```python
from build123d import *

# Parameters (mm, degrees)
SKETCH1_R           = 49.276
BOSS_EXTRUDE1_DEPTH = 9.525
SKETCH2_R           = 47.498
BOSS_EXTRUDE2_DEPTH = 3.175
SKETCH5_R           = 3.175
SKETCH5_R_2         = 1.143
SKETCH5_R_3         = 4.191
SKETCH5_R_4         = 2.54
CUT_EXTRUDE1_DEPTH  = 71.834584434


with BuildPart() as part:
    # Sketch1 → Boss-Extrude1 (new body)
    with BuildSketch(Plane(origin=(0, 0, 0), x_dir=(1, 0, 0), z_dir=(0, 1, 0))):
        with Locations(Location((0, 0, 0), (0, 0, 270))):
            Circle(SKETCH1_R)
    extrude(amount=-BOSS_EXTRUDE1_DEPTH)

    # Sketch2 → Boss-Extrude2 (add)
    with BuildSketch(Plane.XZ.offset(9.525)):
        with Locations(Location((0, 0, 0), (0, 0, 270))):
            Circle(SKETCH2_R)
    extrude(amount=BOSS_EXTRUDE2_DEPTH)

    # Sketch5 → Cut-Extrude1 (cut, through all)
    with BuildSketch(Plane(origin=(0, 0, 0), x_dir=(1, 0, 0), z_dir=(0, 1, 0))):
        with Locations(Location((0, 0, 0), (0, 0, 270))):
            Circle(SKETCH5_R)
        with Locations(Location((0, 29.21, 0), (0, 0, 270))):
            Circle(SKETCH5_R_2)
        with Locations(Location((0, -29.21, 0), (0, 0, 270))):
            Circle(SKETCH5_R_2)
        with Locations(Location((-24.384, 21.59, 0), (0, 0, 270))):
            Circle(SKETCH5_R_3)
        with Locations(Location((-28.448, 6.858, 0), (0, 0, 270))):
            Circle(SKETCH5_R_4)
        with Locations(Location((-26.162, -12.954, 0), (0, 0, 270))):
            Circle(SKETCH5_R)
        with Locations(Location((26.162, -19.812, 0), (0, 0, 270))):
            Circle(SKETCH5_R_3)
        with Locations(Location((28.702, -4.826, 0), (0, 0, 270))):
            Circle(SKETCH5_R_4)
        with Locations(Location((24.13, 16.51, 0), (0, 0, 270))):
            Circle(SKETCH5_R)
    extrude(amount=-CUT_EXTRUDE1_DEPTH, mode=Mode.SUBTRACT)


solid = part.part
```
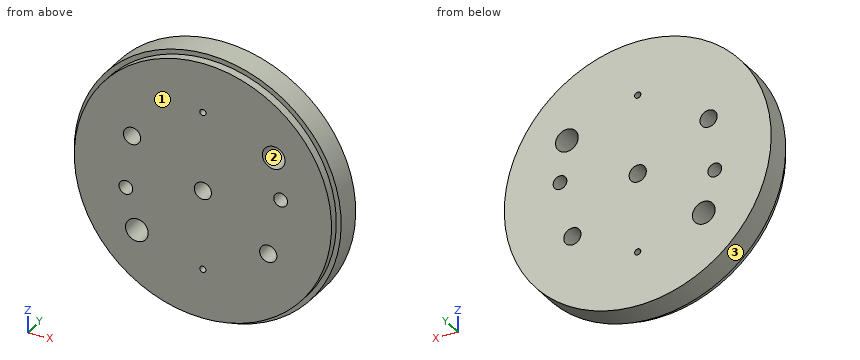
Verification items for the finished model (mm, model axes). Face numbers are marked on the shaded views. Give positions to 0.01 mm unless a question says otherwise; leave off trailing zeros. Order: outer loops, then holes, each group sorted by start corner. A loop starts at its lowest first (then second) coordinate and runs counter-clockwise, first axis right, second up. Notation, with made-up numbers: (-22, 35) -> (31, 35) arc R11 ccw to (31, 55) -> close; hole circle Ø4 at (38.5, 12.5). An arc over 180 degrees is marked (long way). One line per item, written item: value.
(1) Sectioned sample at B-B on y = -7.5. Count the separate pieces of the cut face and the enclosed holes in it, then the cut area to 3 significant figures.
Final values:
separate pieces: 1
enclosed holes: 9
area: 7,370 mm^2
(2) Gauge pin test, flat ends, axial feed: pin 1 (4 mm diameter, centred on x = 39, y = -4.5, fed in from +Z); pin 2 (1.5 mm diameter, centred on x = -28.5, y = -10, fed in from +Z); pin 3 (6 mm diameter, centred on x = 29, y = -6.5, fed in from +Z). Record the tip position at first contact, or that the pin passes through.
Final values:
pin 1: z = 32.54
pin 2: z = 40.6
pin 3: z = 41.86
(3) Sectioned sample at C-C on x = 24.13. Record the cut outline in (y, z) (3 decimals), then the cut area to 4 significant figures.
Final values:
outline: (-12.7, -40.912) -> (-9.525, -40.912) -> (-9.525, -42.964) -> (0, -42.964) -> (0, -19.685) -> (-12.7, -19.685) -> close; (-12.7, -13.335) -> (0, -13.335) -> (0, 16.147) -> (-12.7, 16.147) -> close; (-12.7, 23.477) -> (0, 23.477) -> (0, 42.964) -> (-9.525, 42.964) -> (-9.525, 40.912) -> (-12.7, 40.912) -> close
area: 904.5 mm^2
(4) Draft check along X on the marked faces 1, 2 and 3. Enter one of: pulls with the +X half, pulls with the -X half, needs draft (parallel to the pull), parting line crosses it, or undercut.
Final values:
face 1: needs draft
face 2: undercut
face 3: parting line crosses it
(5) Scan lines: line 1 along Y through (x, z) = (15, 45.5) (3 decimals); line 2 along Z through (x, y) = (-25, -2.25); line 3 along X through (y, z) = (-2.25, 22). Record each from-to range of solid material in increasing order. Write a range as [from, to].
Final values:
line 1: [-9.525, 0]
line 2: [-42.46, -25.74], [-17.44, 10], [15.91, 42.46]
line 3: [-44.09, 22.59], [29.74, 44.09]
(6) Sectioned sample at D-D on x = -35.5. Record the cut outline in (y, z) (3 decimals).
Final values:
outline: (-12.7, -31.556) -> (-9.525, -31.556) -> (-9.525, -34.174) -> (0, -34.174) -> (0, 34.174) -> (-9.525, 34.174) -> (-9.525, 31.556) -> (-12.7, 31.556) -> close
(7) Sectioned sample at A-A on z = 0. Record the cut outline in (x, y) (3 decimals), then the cut area to 3 significant figures.
Final values:
outline: (-49.276, -9.525) -> (-47.498, -9.525) -> (-47.498, -12.7) -> (-3.175, -12.7) -> (-3.175, 0) -> (-49.276, 0) -> close; (3.175, -12.7) -> (47.498, -12.7) -> (47.498, -9.525) -> (49.276, -9.525) -> (49.276, 0) -> (3.175, 0) -> close
area: 1,160 mm^2
